from build123d import *

# Parameters (mm, degrees)
F1_DEPTH = 76
F3_DEPTH = 7.5


with BuildPart() as f1:
    # F0 (on Top) → F1 (new body)
    with BuildSketch(Plane.XY):
        with BuildLine():
            Line((0, 4), (8.774964, 4))
            ThreePointArc((8.774964, 4), (-9, 2), (8.774964, 0))
            Line((8.774964, 0), (0, 0))
            Line((0, 0), (0, 2))
            Line((0, 2), (0, 4))
        make_face()
    extrude(amount=F1_DEPTH)

    # F2 (on face) → F3 (join)
    with BuildSketch(Plane.YZ):
        with BuildLine():
            Line((2, 54.45), (2, 53.2))
            Line((2, 53.2), (2, 51.95))
            ThreePointArc((2, 51.95), (2.883883, 52.316117), (3.25, 53.2))
            ThreePointArc((3.25, 53.2), (2.883883, 54.083883), (2, 54.45))
        make_face()
        with BuildLine():
            Line((2, 51.95), (2, 53.2))
            Line((2, 53.2), (2, 54.45))
            ThreePointArc((2, 54.45), (0.75, 53.2), (2, 51.95))
        make_face()
        with BuildLine():
            ThreePointArc((3.25, 22.8), (2.883883, 23.683883), (2, 24.05))
            Line((2, 24.05), (2, 22.8))
            Line((2, 22.8), (2, 21.55))
            ThreePointArc((2, 21.55), (2.883883, 21.916117), (3.25, 22.8))
        make_face()
        with BuildLine():
            Line((2, 22.8), (2, 24.05))
            ThreePointArc((2, 24.05), (0.75, 22.8), (2, 21.55))
            Line((2, 21.55), (2, 22.8))
        make_face()
        with BuildLine():
            ThreePointArc((3.25, 38), (2.883883, 38.883883), (2, 39.25))
            Line((2, 39.25), (2, 38))
            Line((2, 38), (2, 36.75))
            ThreePointArc((2, 36.75), (2.883883, 37.116117), (3.25, 38))
        make_face()
        with BuildLine():
            Line((2, 38), (2, 39.25))
            ThreePointArc((2, 39.25), (0.75, 38), (2, 36.75))
            Line((2, 36.75), (2, 38))
        make_face()
    extrude(amount=F3_DEPTH)


solid = f1.part
Geometry check sheet. Reference: the model listing, model coordinates, mm. A direction names the side the tool comes from. Round coordinates to 2 decimals unless told otherwise and drop trailing zeros. Loops run counter-clockwise (first coordinate to the right, second up) from the corner with the lowest first, then second, coordinate; pieces in that order, holes last. Notation, with made-up numbers: (85, 89) -> (132, 89) arc R19 cw to (132, 124) -> close; hole circle Ø3 at (54.5, -26.75). An arc over 180 degrees is marked (long way). Answer as a JSON object with one key per item and string values. Group by question number.
Item 1: Thickness scan on line 1 along Y through (x, z) = (7, 38); line 2 along Y through (x, z) = (6.75, 5.5); line 3 along X through (y, z) = (2.25, 36). Record the ranges inside material, lowest first.
Item 2: Cross-section at A-A, the plane x = 4.75. Record the cut outline in (y, z).
Item 3: Depth check by flat-ended pin: pin 1 Ø3 at (y, z) = (6, 63.5) entering from -X; pin 2 Ø2.5 at (y, z) = (1.5, 23) entering from +X; pin 3 Ø1.5 at (y, z) = (-5, 59) entering from +X. Enter the tip coordinate at first touch or a pass-through.
Item 4: Cross-section at C-C, the plane y = -1.5. Record the cut outline in (x, z).
Item 5: Set-up check for faces 1 (the face through (4, 4, 37)), 2 (the face through (0, 3, 37)), 3 (the face through (-0.2, 2.1, 76)): record each of +Z, -Z, +X, -X, +Y, -Y from which the full face is reachable in a straight line by a thin tool's end or side.
Item 6: Release check for a two-part mould opening along Y. For faces 4 (the face through (4, 0, 37)), 5 (the face through (-0.2, 2.1, 0)), 6 (the face through (-9, 2, 37)) record: pulls with the +Y half, pulls with the -Y half, needs draft (parallel to the pull), parting line crosses it, or undercut.
Item 7: Cross-section at B-B, the plane z = 26.5. Record the cut outline in (x, y), plus the area to 3 significant figures.
Determined:
{
 "1": {"line 1": "y = -3.66 to 0, 0.75 to 3.25, 4 to 7.66", "line 2": "y = -3.95 to 0, 4 to 7.95", "line 3": "x = -9 to 0"},
 "2": {"outline": "(-5.64, 0) -> (0, 0) -> (0, 76) -> (-5.64, 76) -> close; (2, 21.55) arc R1.25 ccw to (3.25, 22.8) arc R1.25 ccw to (2, 24.05) arc R1.25 ccw to start; (2, 36.75) arc R1.25 ccw to (3.25, 38) arc R1.25 ccw to (2, 39.25) arc R1.25 ccw to start; (2, 51.95) arc R1.25 ccw to (3.25, 53.2) arc R1.25 ccw to (2, 54.45) arc R1.25 ccw to start; (4, 0) -> (9.64, 0) -> (9.64, 76) -> (4, 76) -> close"},
 "3": {"pin 1": "stops at x = -8.65", "pin 2": "stops at x = 7.5", "pin 3": "stops at x = 6.48"},
 "4": {"outline": "(-8.29, 0) -> (8.29, 0) -> (8.29, 76) -> (-8.29, 76) -> close"},
 "5": {"face 1": "+Z, -Z, +X", "face 2": "+X", "face 3": "+Z, +X, -X, +Y, -Y"},
 "6": {"face 4": "undercut", "face 5": "needs draft", "face 6": "parting line crosses it"},
 "7": {"outline": "(0, 0) -> (0, 4) -> (8.77, 4) arc R9 ccw (long way) to (8.77, 0) -> close", "area": "219 mm²"}
}
